from build123d import *

# Parameters (mm, degrees)
F0_R     = 11.5
F1_DEPTH = 3
F2_R     = 4
F3_DEPTH = 5.5
F4_R     = 6
F5_DEPTH = 3.5
F6_SIZE  = 2
F7_R     = 0.5


with BuildPart() as f1:
    # F0 (on Top) → F1 (new body)
    with BuildSketch(Plane.XY):
        Circle(F0_R)
    extrude(amount=F1_DEPTH)

    # F2 (on face) → F3 (join)
    with BuildSketch(Plane(origin=(0, 0, 0), x_dir=(1, 0, 0), z_dir=(0, 0, -1))):
        Circle(F2_R)
    extrude(amount=F3_DEPTH)

    # F4 (on face) → F5 (join)
    with BuildSketch(Plane(origin=(0, 0, 0), x_dir=(1, 0, 0), z_dir=(0, 0, -1))):
        Circle(F4_R)
    extrude(amount=F5_DEPTH)

    # F6
    f6_edges = [f1.edges().sort_by_distance(p)[0] for p in [
        (-11.5, 0, 3),
    ]]
    chamfer(f6_edges, length=F6_SIZE)

    # F7
    f7_edges = [f1.edges().sort_by_distance(p)[0] for p in [
        (-6, 0, -3.5),
        (-4, 0, -5.5),
        (-11.5, 0, 0),
    ]]
    fillet(f7_edges, radius=F7_R)


solid = f1.part
For this review, take the finished solid that the model builds, in its own axes (mm). A direction names the side the tool comes from. Round coordinates to 2 decimals unless told otherwise and drop trailing zeros. Write each loop counter-clockwise with the first axis right and the second up, starting at its lowest first coordinate (ties: lowest second). Pieces come first, ordered by that corner, then holes. Notation, with made-up numbers: M -8,37 L -1,37 A23 cw -1,54 Z; hole C -37,-30.5 d2. An arc over 180 degrees is marked long. Write item = value, one per line. Start each with the question number.
(1) We need section C-C (z = -1.5). Give the boundary of the cut face in (x, y).
(2) For faces 1 (the face through (0, 0, -5.5)), 2 (the face through (-6, 0, -1)), list the 3-axis set-ups (+Z, -Z, +X, -X, +Y, -Y) from which the entire face can be reached by the end or side of a thin tool; tool diameter is ignored.
(3) For line 1 along Z through (x, y) = (-9.25, 0.25); line 2 along X through (y, z) = (0, -0.5); line 3 along X through (y, z) = (0, -4.25), list the stretches that pass through material, from the lowest coordinate up.
(4) Clearance check with flat-ended pins moving along their axes: pin 1 Ø1 at (x, y) = (-8, 4) entering from -Z; pin 2 Ø5 at (y, z) = (7.5, 0) entering from +X; pin 3 Ø4 at (x, z) = (-2, -2.5) entering from -Y. State where each tip first meets the part, or that it passes through.
(5) We need section A-A (y = 0). Give the boundary of the cut face in (x, z).
Results found:
q1.outline = C 0,0 d12
q2.face_1 = -Z, +X, -X, +Y, -Y
q2.face_2 = -Z
q3.line_1 = 0 to 3
q3.line_2 = -6 to 6
q3.line_3 = -4 to 4
q4.pin_1 = 0
q4.pin_2 = 10.33
q4.pin_3 = -6
q5.outline = M -11.5,0.5 A0.5 ccw -11,0 L -6,0 L -6,-3 A0.5 ccw -5.5,-3.5 L -4,-3.5 L -4,-5 A0.5 ccw -3.5,-5.5 L 3.5,-5.5 A0.5 ccw 4,-5 L 4,-3.5 L 5.5,-3.5 A0.5 ccw 6,-3 L 6,0 L 11,0 A0.5 ccw 11.5,0.5 L 11.5,1 L 9.5,3 L -9.5,3 L -11.5,1 Z
